from build123d import *

# Parameters (mm, degrees)
EXTRUDE_1_DEPTH     = 4.2
EXTRUDE_2_DEPTH     = 12.8
SKETCH_3_R          = 1
CUT_EXTRUDE_1_DEPTH = 10
SKETCH_5_W          = 1
SKETCH_5_H          = 2.7
EXTRUDE_3_DEPTH     = 12.8


with BuildPart() as part:
    # 草图1 → 凸台-拉伸1 (new body)
    with BuildSketch(Plane.XY):
        with BuildLine():
            Line((6.01, 10.345093063), (6.01, -43.654906937))
            ThreePointArc((6.01, -43.654906937), (0, -49.664906937), (-6.01, -43.654906937))
            Line((-6.01, -43.654906937), (-6.01, 10.345093063))
            ThreePointArc((-6.01, 10.345093063), (0, 16.355093063), (6.01, 10.345093063))
        make_face()
        with BuildLine():
            Line((3.51, 10.345093063), (3.51, -43.654906937))
            ThreePointArc((3.51, -43.654906937), (0, -47.164906937), (-3.51, -43.654906937))
            Line((-3.51, -43.654906937), (-3.51, 10.345093063))
            ThreePointArc((-3.51, 10.345093063), (0, 13.855093063), (3.51, 10.345093063))
        make_face(mode=Mode.SUBTRACT)
    extrude(amount=EXTRUDE_1_DEPTH)

    # 草图2 → 凸台-拉伸2 (add)
    with BuildSketch(Plane.ZY.offset(6.01)):
        Polygon((4.2, -16.654906937), (4.2, -8.154906937), (-2.6, -8.154906937), (-2.6, -10.154906937), (2.2, -10.154906937), (2.2, -17.154906937), (-2.6, -17.154906937), (-2.6, -19.154906937), (4.2, -19.154906937), align=None)
    extrude(amount=EXTRUDE_2_DEPTH)

    # 草图3 → 切除-拉伸1 (cut)
    with BuildSketch(Plane(origin=(0, 0, 2.2), x_dir=(-1, 0, 0), z_dir=(0, 0, -1))):
        with Locations((11.01, -13.654906937)):
            Circle(SKETCH_3_R)
    extrude(amount=-CUT_EXTRUDE_1_DEPTH, mode=Mode.SUBTRACT)

    # 草图5 → 凸台-拉伸3 (add, through all)
    with BuildSketch(Plane(origin=(-6.01, 0, 0), x_dir=(0, 0, -1), z_dir=(1, 0, 0))):
        with Locations((3.1, -9.504906937)):
            Rectangle(SKETCH_5_W, SKETCH_5_H)
        with Locations((3.1, -17.804906937)):
            Rectangle(SKETCH_5_W, SKETCH_5_H)
    extrude(amount=-EXTRUDE_3_DEPTH)


solid = part.part
Read the model definition and answer for the solid it produces. Units are mm, in the model's axes. A direction names the side the tool comes from. Give positions to 0.01 mm unless a question says otherwise; leave off trailing zeros. Write each loop counter-clockwise with the first axis right and the second up, starting at its lowest first coordinate (ties: lowest second). Pieces come first, ordered by that corner, then holes. Notation, with made-up numbers: (41.25, 63) - (88.25, 63) arc R30 ccw to (88.25, 88) - close; hole circle Ø1 at (-13, -8.5). An arc over 180 degrees is marked (long way). Return JSON: item names as keys, results as strings.
Q1. For a pull along Y with two mould halves and no side action, classify faces 5 (the face through (-10.27, -12.98, 3.19)), 6 (the face through (-6.01, -32, 2)), 7 (the face through (-0.077, 13.854, 2.071)), 8 (the face through (0.132, -49.663, 2.071)) as released by +Y, released by -Y, zero draft, split by the parting line, or undercut.
Reply:
{"face 5": "undercut", "face 6": "zero draft", "face 7": "undercut", "face 8": "released by -Y"}
Q2. A cutting plane is placed at D-D, the plane x = -4.75. Determine the outline of the cut face in (y, z), and give its area (3 significant figures).
Reply:
{"outline": "(-47.34, 0) - (14.03, 0) - (14.03, 4.2) - (-47.34, 4.2) - close", "area": "258 mm²"}
Q3. Given P1, Ø2.5, axis at x = -11.01, y = -13.65, coming from the -Z side; P2, Ø0.8, axis at y = -18, z = -2, coming from the +X side; P3, Ø3, axis at y = -1.5, z = -2, coming from the +X side; P4, Ø2.5, axis at x = -9.5, z = 1, coming from the +Y side, each flat-ended and moving along its own axis, determine where each tip first touches the part or whether it passes through.
Reply:
{"P1": "z = 2.2", "P2": "x = -6.01", "P3": "through", "P4": "y = -8.15"}
Q4. For faces 1 (the face through (0.077, -47.164, 2.071)), 2 (the face through (-6.01, -9, -2)), 3 (the face through (-12, -19.155, 0)), 4 (the face through (-6.01, -14, 1)), determine the directions among +Z, -Z, +X, -X, +Y, -Y from which every point of the face is accessible in a straight line to the end or side of a thin tool.
Reply:
{"face 1": "+Z, -Z", "face 2": "-Z, +X, +Y, -Y", "face 3": "+Z, -Z, -X, -Y", "face 4": "-X"}
Q5. A cutting plane is placed at C-C, the plane x = -9. Determine the outline of the cut face in (y, z), and give its area (3 significant figures).
Reply:
{"outline": "(-19.15, -3.6) - (-16.45, -3.6) - (-16.45, -2.6) - (-17.15, -2.6) - (-17.15, 2.2) - (-10.15, 2.2) - (-10.15, -2.6) - (-10.85, -2.6) - (-10.85, -3.6) - (-8.15, -3.6) - (-8.15, 4.2) - (-19.15, 4.2) - close", "area": "46.6 mm²"}
Q6. A cutting plane is placed at B-B, the plane y = -28. Determine the outline of the cut face in (x, z).
Reply:
{"outline": "(-6.01, 0) - (-3.51, 0) - (-3.51, 4.2) - (-6.01, 4.2) - close; (3.51, 0) - (6.01, 0) - (6.01, 4.2) - (3.51, 4.2) - close"}
Q7. A cutting plane is placed at A-A, the plane x = 0. Determine the outline of the cut face in (y, z).
Reply:
{"outline": "(-49.66, 0) - (-47.16, 0) - (-47.16, 4.2) - (-49.66, 4.2) - close; (13.86, 0) - (16.36, 0) - (16.36, 4.2) - (13.86, 4.2) - close"}
Q8. Consider line 1 along Y through (x, z) = (-11.01, 3.3); line 2 along X through (y, z) = (10, 1.75); line 3 along Y through (x, z) = (-16, 1.75). Determine where each line is inside the solid, lowest interval first. Write a range as [from, to].
Reply:
{"line 1": "[-19.15, -14.65], [-12.65, -8.15]", "line 2": "[-6.01, -3.51], [3.51, 6.01]", "line 3": "[-19.15, -17.15], [-10.15, -8.15]"}
